from build123d import *

# Parameters (mm, degrees)
BOSS_EXTRUDE1_DEPTH   = 1.6
F_4_CLEARANCE_HOLE1_D = 3.2639
SKETCH4_W             = 14.7828
SKETCH4_H             = 13.5382
BOSS_EXTRUDE2_DEPTH   = 8.1534


with BuildPart() as part:
    # Sketch1 → Boss-Extrude1 (new body)
    with BuildSketch(Plane(origin=(0, 0, 0), x_dir=(1, 0, 0), z_dir=(0, 1, 0))):
        with BuildLine():
            Line((23.3172, -30.2006), (23.3172, -23.0124))
            ThreePointArc((23.3172, -23.0124), (24.384, -21.9456), (25.4508, -23.0124))
            Line((25.4508, -23.0124), (25.4508, -30.2006))
            Line((25.4508, -30.2006), (32.5882, -30.2006))
            Line((32.5882, -30.2006), (32.5882, 30.2006))
            Line((32.5882, 30.2006), (-32.5882, 30.2006))
            Line((-32.5882, 30.2006), (-32.5882, -26.0096))
            Line((-32.5882, -26.0096), (-17.6276, -26.0096))
            Line((-17.6276, -26.0096), (-17.6276, -19.7292))
            ThreePointArc((-17.6276, -19.7292), (-17.041813562, -18.314986438), (-15.6276, -17.7292))
            Line((-15.6276, -17.7292), (-1.365, -17.7292))
            ThreePointArc((-1.365, -17.7292), (0.049213562, -18.314986438), (0.635, -19.7292))
            Line((0.635, -19.7292), (0.635, -25.7556))
            Line((0.635, -25.7556), (8.5852, -25.7556))
            Line((8.5852, -25.7556), (8.5852, -18.8976))
            ThreePointArc((8.5852, -18.8976), (10.4902, -16.9926), (12.3952, -18.8976))
            Line((12.3952, -18.8976), (12.3952, -30.2006))
            Line((12.3952, -30.2006), (23.3172, -30.2006))
        make_face()
    extrude(amount=BOSS_EXTRUDE1_DEPTH)

    # #4 Clearance Hole1 (through all)
    with Locations(Plane(origin=(0, 1.6, 0), x_dir=(1, 0, 0), z_dir=(0, 1, 0))):
        with Locations((-24.6126, 25.7302), (-24.6126, -21.5392)):
            Hole(F_4_CLEARANCE_HOLE1_D / 2)

    # Sketch4 → Boss-Extrude2 (add)
    with BuildSketch(Plane(origin=(0, 1.6, 0), x_dir=(1, 0, 0), z_dir=(0, 1, 0))):
        with Locations((-27.7368, 13.2588)):
            Rectangle(SKETCH4_W, SKETCH4_H)
        with Locations((-27.7368, -9.0678)):
            Rectangle(SKETCH4_W, SKETCH4_H)
    extrude(amount=BOSS_EXTRUDE2_DEPTH)


solid = part.part
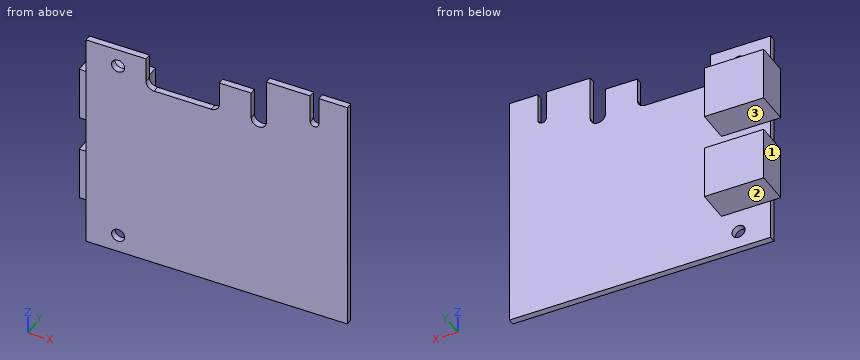
Here's how the part is built. I have some questions about the finished solid (model axes, mm). Face numbers are marked on the shaded views. Round coordinates to 2 decimals unless told otherwise and drop trailing zeros. Loops run counter-clockwise (first coordinate to the right, second up) from the corner with the lowest first, then second, coordinate; pieces in that order, holes last.
1. If we section it at B-B on x = -24: Write out the boundary of the cut face in (y, z), plus the area to 3 significant figures.
Answer list:
outline: (0, -30.2) - (1.6, -30.2) - (1.6, -27.24) - (0, -27.24) - close; (0, -24.22) - (1.6, -24.22) - (1.6, -20.03) - (9.75, -20.03) - (9.75, -6.49) - (1.6, -6.49) - (1.6, 2.3) - (9.75, 2.3) - (9.75, 15.84) - (1.6, 15.84) - (1.6, 20.03) - (0, 20.03) - close; (0, 23.05) - (1.6, 23.05) - (1.6, 26.01) - (0, 26.01) - close
area: 301 mm2
2. If we section it at A-A on y = 7.75: Write out the boundary of the cut face in (x, z), plus the area to 3 significant figures.
Answer list:
outline: (-35.13, -20.03) - (-20.35, -20.03) - (-20.35, -6.49) - (-35.13, -6.49) - close; (-35.13, 2.3) - (-20.35, 2.3) - (-20.35, 15.84) - (-35.13, 15.84) - close
area: 400 mm2
3. If we section it at D-D on x = -13: Write out the boundary of the cut face in (y, z), plus the area to 3 significant figures.
Answer list:
outline: (0, -30.2) - (1.6, -30.2) - (1.6, 17.73) - (0, 17.73) - close
area: 76.7 mm2
4. If I drill on line 1 along Z through (x, y) = (-22, 4.5); line 2 along Y through (x, z) = (-1.5, -6.5); line 3 along X through (y, z) = (4.25, 8.5), over which ranges is the centre line in solid material (lowest first)?
Answer list:
line 1: z = -20.03 to -6.49, 2.3 to 15.84
line 2: y = 0 to 1.6
line 3: x = -35.13 to -20.35
5. If we section it at C-C on z = -9: Write out the boundary of the cut face in (x, y), plus the area to 3 significant figures.
Answer list:
outline: (-35.13, 1.6) - (-32.59, 1.6) - (-32.59, 0) - (32.59, 0) - (32.59, 1.6) - (-20.35, 1.6) - (-20.35, 9.75) - (-35.13, 9.75) - close
area: 225 mm2
6. For P1, Ø1.3, axis at x = -33.5, z = 6.5, coming from the -Y side; P2, Ø2, axis at x = -22, y = 5.5, coming from the +Z side; P3, Ø0.5, axis at y = 1, z = 25.5, coming from the -X side; P4, Ø1.5, axis at x = 20, y = 3, coming from the +Z side, each with a flat end and sliding along its axis, tell me the tip position at first contact or that it passes through.
Answer list:
P1: stops at y = 1.6
P2: stops at z = 15.84
P3: stops at x = -32.59
P4: passes through
7. We'd pull the mould along Z, two halves only. Please class the marked faces 1, 2 and 3: +Z half, -Z half, draft (parallel to the pull), parting line (faces both ways), or undercut.
Answer list:
face 1: draft
face 2: -Z half
face 3: undercut
